```python
from build123d import *

# Parameters (mm, degrees)
SKETCH2_R           = 6.35
SKETCH3_R           = 19.05
SKETCH4_R           = 3.175
BOSS_EXTRUDE1_DEPTH = 19.05
DOME1_FACE_RADIUS   = 19.05
DOME1_HEIGHT        = 25.4


with BuildPart() as part:
    # Sketch2 → Loft1 section 0
    with BuildSketch(Plane(origin=(0, 0, 0), x_dir=(1, 0, 0), z_dir=(0, 1, 0))):
        Circle(SKETCH2_R)
    # Sketch3 → Loft1 section 1
    with BuildSketch(Plane(origin=(0, 76.2, 0), x_dir=(1, 0, 0), z_dir=(0, 1, 0))):
        Circle(SKETCH3_R)
    loft()

    # Sketch4 → Boss-Extrude1 (add)
    with BuildSketch(Plane.XZ):
        with Locations(Location((0, 0, 0), (0, 0, 90))):
            Circle(SKETCH4_R)
    extrude(amount=BOSS_EXTRUDE1_DEPTH)

    # Dome1: a dome of height H over a round flat face of radius A is a cap of a sphere of radius (A * A + H * H) / (2 * H)
    dome1_r = (DOME1_FACE_RADIUS * DOME1_FACE_RADIUS + DOME1_HEIGHT * DOME1_HEIGHT) / (2 * DOME1_HEIGHT)
    dome1_base = Plane((0, 76.2, 0), z_dir=(0, 1, 0))
    with Locations(dome1_base.offset(DOME1_HEIGHT - dome1_r)):
        dome1_ball = Sphere(dome1_r, mode=Mode.PRIVATE)
    add(split(dome1_ball, bisect_by=dome1_base, keep=Keep.TOP, mode=Mode.PRIVATE))


solid = part.part
```
The model under review builds one solid part; all positions refer to its coordinate system, in mm. A direction names the side the tool comes from. Round coordinates to 2 decimals unless told otherwise and drop trailing zeros. Write each loop counter-clockwise with the first axis right and the second up, starting at its lowest first coordinate (ties: lowest second). Pieces come first, ordered by that corner, then holes. Notation, with made-up numbers: (25, 68.25) - (37, 68.25) arc R11 cw to (37, 89.25) - close; hole circle Ø10 at (25, 40.25). An arc over 180 degrees is marked (long way). Answer as CSV lines item,"result". Start each with the question number.
(1) We need section C-C on y = 87. State the section outline as (x, z) points, plus the area to 3 significant figures.
(2) For pin 1 Ø10 at (x, y) = (1, 71) entering from -Z; pin 2 Ø5 at (x, z) = (-8.5, 5.5) entering from +Y; pin 3 Ø5 at (x, y) = (-12, 17) entering from -Z; pin 4 Ø1.5 at (y, z) = (39.5, -12.5) entering from -X, all flat-tipped, find the tip position at first contact; note any pin that passes through.
(3) We need section B-B on y = 61.5. State the section outline as (x, z) points, plus the area to 3 significant figures.
(4) For faces 1 (the flat face through (0, -19.05, 0)), 2 (the cylindrical face through (1.93, -9.39, -2.52)), list the 3-axis set-ups (+Z, -Z, +X, -X, +Y, -Y) from which the entire face can be reached by the end or side of a thin tool; tool diameter is ignored.
(5) To check wall thickness, follow line 1 (X direction, y = 89.5, z = 3); line 2 (Z direction, x = -0.5, y = 20.5); line 3 (Z direction, x = -11.5, y = 62). State the ranges of each line that lie inside material, in increasing order.
Worked answers:
1,outline,"circle Ø38.28 at (0, 0)"
1,area,"1,150 mm²"
2,pin 1,"z = -19.01"
2,pin 2,"y = 100.08"
2,pin 3,"through"
2,pin 4,"x = -5.43"
3,outline,"circle Ø33.2 at (0, 0)"
3,area,"866 mm²"
4,face 1,"+Z, -Z, +X, -X, -Y"
4,face 2,"-Y"
5,line 1,"-18.02 to 18.02"
5,line 2,"-9.75 to 9.75"
5,line 3,"-12.09 to 12.09"
